```python
from build123d import *

# Parameters (mm, degrees)
F1_DEPTH  = 800
F1_TAPER  = 8
F2_T      = -1.6
F3_R      = 247.5
F4_DEPTH  = 25
F6_DEPTH  = 25
F8_DEPTH  = 25
F10_DEPTH = 25
F12_DEPTH = 25
F14_DEPTH = 25
F16_DEPTH = 25


with BuildPart() as f1:
    # F0 (on Top) → F1 (new body)
    with BuildSketch(Plane.XY):
        Polygon((172.0503802185, 298), (-172.0503802185, 298), (-344.100760437, 0), (-172.0503802185, -298), (172.0503802185, -298), (344.100760437, 0), align=None)
    extrude(amount=F1_DEPTH, taper=F1_TAPER)

    # F2
    f2_openings = [f1.faces().sort_by_distance(p)[0] for p in [
        (0, 0, 800),
    ]]
    offset(amount=F2_T, openings=f2_openings)

    # F3 (on face) → F4 (cut)
    with BuildSketch(Plane.XY):
        Circle(F3_R)
    extrude(amount=F4_DEPTH, mode=Mode.SUBTRACT)

    # F5 (on face) → F6 (cut)
    with BuildSketch(Plane(origin=(0, -292.2279926948, 41.0699660167), x_dir=(1, 0, 0), z_dir=(0, -0.9902680687, 0.139173101))):
        Polygon((-86.8341790619, 744.3884739288), (-148.2117384586, -19.4735840861), (148.2117384586, -19.4735840861), (86.8341790619, 744.3884739288), align=None)
    extrude(amount=-F6_DEPTH, mode=Mode.SUBTRACT)

    # F7 (on face) → F8 (cut)
    with BuildSketch(Plane(origin=(-253.0768653706, -146.1139963474, 41.0699660167), x_dir=(0.4887402152, -0.8688166021, -0.0793140218), z_dir=(-0.8575973041, -0.4951340344, 0.139173101))):
        Polygon((-146.1758796985, 735.0421667944), (-146.1758796985, -31.2818172178), (149.2952941729, -7.540227576), (26.934543851, 748.9518710297), align=None)
    extrude(amount=-F8_DEPTH, mode=Mode.SUBTRACT)

    # F9 (on face) → F10 (cut)
    with BuildSketch(Plane(origin=(-253.0768653706, 146.1139963474, 41.0699660167), x_dir=(-0.4887402152, -0.8688166021, 0.0793140218), z_dir=(-0.8575973041, 0.4951340344, 0.139173101))):
        Polygon((146.1758796985, 735.0421667944), (-26.934543851, 748.9518710297), (-149.2952941729, -7.540227576), (146.1758796985, -31.2818172178), align=None)
    extrude(amount=-F10_DEPTH, mode=Mode.SUBTRACT)

    # F11 (on face) → F12 (cut)
    with BuildSketch(Plane(origin=(0, 292.2279926948, 41.0699660167), x_dir=(-1, 0, 0), z_dir=(0, 0.9902680687, 0.139173101))):
        Polygon((-148.2117384586, -19.4735840861), (148.2117384586, -19.4735840861), (86.8341790619, 744.3884739288), (-86.8341790619, 744.3884739288), align=None)
    extrude(amount=-F12_DEPTH, mode=Mode.SUBTRACT)

    # F13 (on face) → F14 (cut)
    with BuildSketch(Plane(origin=(253.0768653706, 146.1139963474, 41.0699660167), x_dir=(-0.4887402152, 0.8688166021, -0.0793140218), z_dir=(0.8575973041, 0.4951340344, 0.139173101))):
        Polygon((26.934543851, 748.9518710297), (-146.1758796985, 735.0421667944), (-146.1758796985, -31.2818172178), (149.2952941729, -7.540227576), align=None)
    extrude(amount=-F14_DEPTH, mode=Mode.SUBTRACT)

    # F15 (on face) → F16 (cut)
    with BuildSketch(Plane(origin=(253.0768653706, -146.1139963474, 41.0699660167), x_dir=(0.4887402152, 0.8688166021, 0.0793140218), z_dir=(0.8575973041, -0.4951340344, 0.139173101))):
        Polygon((-26.934543851, 748.9518710297), (-149.2952941729, -7.540227576), (146.1758796985, -31.2818172178), (146.1758796985, 735.0421667944), align=None)
    extrude(amount=-F16_DEPTH, mode=Mode.SUBTRACT)


solid = f1.part
```
Work out the finished part from the listing and answer in its coordinate system (mm). A direction names the side the tool comes from. Coordinates: 2 decimals unless noted, no trailing zeros. Loops run counter-clockwise (first coordinate to the right, second up) from the corner with the lowest first, then second, coordinate; pieces in that order, holes last. Notation, with made-up numbers: (48, -36.5) - (61, -36.5) arc R21 cw to (61, -2.5) - close; hole circle Ø11 at (-3, 56). An arc over 180 degrees is marked (long way). Use a Markdown table: item, result.
Item 1: For faces 1 (the flat face through (149.523, -221.535, 405.185)), 2 (the flat face through (266.617, 18.723, 405.185)), 3 (the flat face through (125.86, 248.63, 339.8)), determine the directions among +Z, -Z, +X, -X, +Y, -Y from which every point of the face is accessible in a straight line to the end or side of a thin tool.
Evaluation:
| item | result |
|---|---|
| face 1 | +X |
| face 2 | +Y |
| face 3 | none |
Item 2: The mould has two halves that part along X. Classify faces 4 (the flat face through (-162.073, -94.977, 778.104)), 5 (the flat face through (205.3, -12.9, 800)), 6 (the flat face through (-152.39, 233.31, 339.8)): +X half, -X half, draft (parallel to the pull), parting line (faces both ways), or undercut.
Evaluation:
| item | result |
|---|---|
| face 4 | -X half |
| face 5 | draft |
| face 6 | undercut |
Item 3: Consider probe 1 along Y at (x, z) = (0, 1.1); probe 2 along X at (y, z) = (0, 0.9); probe 3 along Y at (x, z) = (0, 1). Determine where each line is inside the solid, lowest interval first. Write a range as from..to.
Evaluation:
| item | result |
|---|---|
| probe 1 | y = -297.85..-247.5, 247.5..297.85 |
| probe 2 | x = -343.95..-247.5, 247.5..343.95 |
| probe 3 | y = -297.86..-247.5, 247.5..297.86 |
Item 4: Find section C-C, the plane x = 269.5. Determine the outline of the cut face in (y, z), and give its area (3 significant figures).
Evaluation:
| item | result |
|---|---|
| outline | (-129.21, 0) - (129.21, 0) - (123.09, 21.79) - (119.92, 21.56) - (125.53, 1.6) - (-125.53, 1.6) - (-119.92, 21.56) - (-123.09, 21.79) - close; (-19.11, 391.7) - (-18.32, 383.02) - (0, 448.2) - (18.32, 383.02) - (19.11, 391.7) - (0, 459.7) - close |
| area | 973 mm2 |
Item 5: Given pin 1 Ø6 at (y, z) = (11, 227) entering from +X; pin 2 Ø3 at (x, z) = (-146, 192) entering from +Y, each flat-ended and moving along its own axis, determine where each tip first touches the part or whether it passes through.
Evaluation:
| item | result |
|---|---|
| pin 1 | stops at x = 302.71 |
| pin 2 | stops at y = 271.23 |
Item 6: Find section D-D, the plane z = 580.5. State how many separate pieces and enclosed holes the cut face has, and give its area (3 significant figures).
Evaluation:
| item | result |
|---|---|
| separate pieces | 6 |
| enclosed holes | 0 |
| area | 419 mm2 |
Item 7: Find section B-B, the plane y = 219.5. Determine the outline of the cut face in (x, z), and give its area (3 significant figures).
Evaluation:
| item | result |
|---|---|
| outline | (-217.37, 0) - (-114.35, 0) - (-114.35, 1.6) - (-215.25, 1.6) - (-212.01, 21.56) - (-213.84, 21.79) - close; (-148.8, 422.55) - (-147.88, 416.69) - (-126.73, 547.06) - (-105.57, 547.06) - (-104.66, 558.56) - (-126.73, 558.56) - close; (104.66, 558.56) - (105.57, 547.06) - (126.73, 547.06) - (147.88, 416.69) - (148.8, 422.55) - (126.73, 558.56) - close; (114.35, 0) - (217.37, 0) - (213.84, 21.79) - (212.01, 21.56) - (215.25, 1.6) - (114.35, 1.6) - close |
| area | 1,400 mm2 |
Item 8: Find section A-A, the plane x = 0. Determine the outline of the cut face in (y, z), and give its area (3 significant figures).
Evaluation:
| item | result |
|---|---|
| outline | (-298, 0) - (-247.5, 0) - (-247.5, 1.6) - (-296.16, 1.6) - (-293.35, 21.56) - (-294.94, 21.79) - close; (-188.63, 778.21) - (-187.04, 777.99) - (-183.95, 800) - (-185.57, 800) - close; (183.95, 800) - (187.04, 777.99) - (188.63, 778.21) - (185.57, 800) - close; (247.5, 0) - (298, 0) - (294.94, 21.79) - (293.35, 21.56) - (296.16, 1.6) - (247.5, 1.6) - close |
| area | 297 mm2 |
